For this review, take the finished solid that the model builds, in its own axes (mm). A direction names the side the tool comes from. Coordinates: 2 decimals unless noted, no trailing zeros. Order: outer loops, then holes, each group sorted by start corner. A loop starts at its lowest first (then second) coordinate and runs counter-clockwise, first axis right, second up. Notation, with made-up numbers: M 80.25,78.25 L 124.25,78.25 A9 ccw 124.25,90.25 Z; hole C -8.75,75 d5. An arc over 180 degrees is marked long. Use one line per item in the form item = value. Start each with the question number.
```python
from build123d import *

# Parameters (mm, degrees)
BOSS_EXTRUDE1_DEPTH = 80


with BuildPart() as part:
    # Sketch1 → Boss-Extrude1 (new body)
    with BuildSketch(Plane(origin=(0, 0, 0), x_dir=(1, 0, 0), z_dir=(0, 1, 0))):
        with BuildLine():
            Line((-79.797325403, -29.387699101), (-65.53287479, -24.605737578))
            ThreePointArc((-65.53287479, -24.605737578), (-61.954038815, -32.583693383), (-57.408519486, -40.053238201))
            Line((-57.408519486, -40.053238201), (-53.307910951, -37.192292615))
            ThreePointArc((-53.307910951, -37.192292615), (-61.629140737, -20.660324585), (-64.953686456, -2.453286719))
            Line((-64.953686456, -2.453286719), (-69.950123876, -2.642001082))
            ThreePointArc((-69.950123876, -2.642001082), (-69.075024078, -11.342003731), (-67.122130527, -19.865034445))
            Line((-67.122130527, -19.865034445), (-81.386581141, -24.646995968))
            Line((-81.386581141, -24.646995968), (-79.797325403, -29.387699101))
        make_face()
    extrude(amount=BOSS_EXTRUDE1_DEPTH)


solid = part.part
```
1. Consider section C-C, the plane z = 36. Write out the cut boundary in (x, y), plus the area to 3 significant figures.
2. The part is to be moulded in two halves that separate along Z. For faces 3 (the cylindrical face through (-69.1, 39.4, 11.2)), 4 (the flat face through (-74.15, 39.44, 22.22)), 5 (the flat face through (-55.387, 39.44, 38.643)), 6 (the flat face through (-67.417, 39.44, 2.546)), say which applies: pulls with the +Z half, pulls with the -Z half, needs draft (parallel to the pull), parting line crosses it, or undercut.
3. Consider section A-A, the plane y = 51. Write out the cut boundary in (x, z).
4. Consider section B-B, the plane x = -74.5. Write out the cut boundary in (y, z), plus the area to 3 significant figures.
5. Tool access review of faces 1 (the flat face through (-66, 0, 21)), 2 (the cylindrical face through (-62, 39.4, 32.5)): name each direction out of +Z, -Z, +X, -X, +Y, -Y from which nothing blocks a thin tool from reaching the whole face with its end or side.
6. For pin 1 Ø10 at (x, y) = (-58.5, 61) entering from +Z; pin 2 Ø12 at (y, z) = (28, 6.5) entering from +X; pin 3 Ø2 at (y, z) = (53.5, 6.5) entering from +X, all flat-tipped, find the tip position at first contact; note any pin that passes through.
7. To check wall thickness, follow line 1 (Z direction, x = -79, y = 62); line 2 (X direction, y = 34.5, z = 13.5); line 3 (Z direction, x = -58.25, y = 3). State the ranges of each line that lie inside material, in increasing order.
Answers follow:
q1.outline = M -60.03,0 L -54.12,0 L -54.12,80 L -60.03,80 Z
q1.area = 473 mm²
q2.face_3 = undercut
q2.face_4 = undercut
q2.face_5 = pulls with the +Z half
q2.face_6 = pulls with the -Z half
q3.outline = M -81.39,24.65 L -67.12,19.87 A70 ccw -69.95,2.64 L -64.95,2.45 A65 cw -53.31,37.19 L -57.41,40.05 A70 ccw -65.53,24.61 L -79.8,29.39 Z
q4.outline = M 0,22.34 L 80,22.34 L 80,27.61 L 0,27.61 Z
q4.area = 422 mm²
q5.face_1 = +Z, -Z, +X, -X, -Y
q5.face_2 = +Z, +Y, -Y
q6.pin_1 = 40.05
q6.pin_2 = -63.79
q6.pin_3 = -64.57
q7.line_1 = 23.85 to 29.12
q7.line_2 = -68.69 to -63.58
q7.line_3 = 28.84 to 38.82
